For this review, take the finished solid that the model builds, in its own axes (mm). Face numbers are marked on the shaded views. A direction names the side the tool comes from. Round coordinates to 2 decimals unless told otherwise and drop trailing zeros. Loops run counter-clockwise (first coordinate to the right, second up) from the corner with the lowest first, then second, coordinate; pieces in that order, holes last.
1. To check wall thickness, follow line 1 along Y through (x, z) = (-10.5, -2); line 2 along X through (y, z) = (0.8, -0.5); line 3 along Z through (x, y) = (-11.25, 0.95). State the ranges of each line that lie inside material, in increasing order.
2. Consider section B-B on x = -6.25. State the section outline as (y, z) points, then the cut area to 3 significant figures.
3. Consider section C-C on x = -0.75. State the section outline as (y, z) points.
4. Tool access review of the marked faces 1 and 2: name each direction out of +Z, -Z, +X, -X, +Y, -Y from which nothing blocks a thin tool from reaching the whole face with its end or side.
5. Consider section A-A on z = -8. State the section outline as (x, y) points, then the cut area to 3 significant figures.
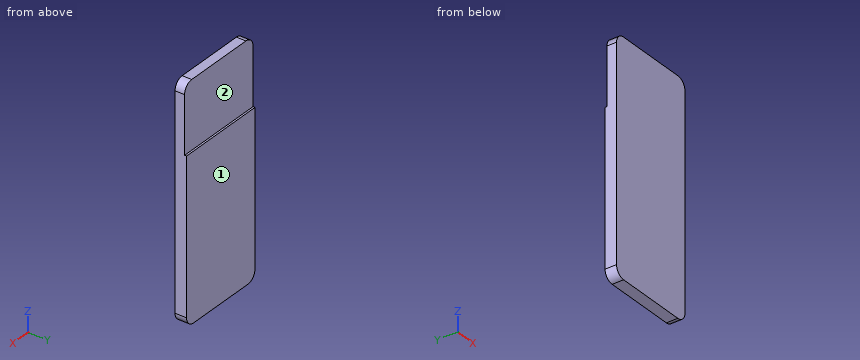
Autodesk Inventor part; units mm, degrees
ref_plane "YZ Plane" through (0, 0, 0) normal (1, 0, 0) x (0, 1, 0)
ref_plane "XZ Plane" through (0, 0, 0) normal (0, 1, 0) x (-1, 0, 0)
ref_plane "XY Plane" through (0, 0, 0) normal (0, 0, 1) x (1, 0, 0)
sketch "Sketch1" plane through (0, 0, 0) normal (0, 1, 0) x (-1, 0, 0)
  line L0 (1.27, 0) -> (10.922, 0)
  line L1 (12.192, -1.27) -> (12.192, -29.21)
  line L2 (10.922, -30.48) -> (1.27, -30.48)
  line L3 (0, -29.21) -> (0, -1.27)
  arc A0 (12.192, -1.27) -> (10.922, 0) centre (10.922, -1.27) ccw
  arc A1 (1.27, 0) -> (0, -1.27) centre (1.27, -1.27) ccw
  arc A2 (0, -29.21) -> (1.27, -30.48) centre (1.27, -29.21) ccw
  arc A3 (10.922, -30.48) -> (12.192, -29.21) centre (10.922, -29.21) ccw
  point P0 (0, 0)
  point P1 (12.192, -30.48)
  point P2 (12.192, 0)
  point P3 (0, -30.48)
  dimension "d0" = 12.192
  dimension "d1" = 30.48
  dimension "d2" = 1.27
extrude "Extrusion1" add sketch "Sketch1" along normal blind 1.524
sketch "Sketch2" plane through (0, 1.524, 0) normal (0, 1, 0) x (1, 0, 0)
  line L0 (0, 1.27) -> (0, 29.21)
  line L1 (-12.192, 0) -> (0, 0)
  line L2 (0, 0) -> (0, 8.89)
  line L3 (0, 8.89) -> (-12.192, 8.89)
  line L4 (-12.192, 8.89) -> (-12.192, 0)
  arc A0 (-12.192, 1.27) -> (-10.922, 0) centre (-10.922, 1.27) ccw
  line L5 (-10.922, 0) -> (-1.27, 0) construction
  point P0 (0, 0)
  dimension "d5" = 8.89
  dimension "d6" = 12.192
  dimension "d7" = 9.652
extrude "Extrusion2" cut sketch "Sketch2" against normal blind 0.254
properties part number "Adafruit-MicroLipoBatteryCharger"
Resolved:
1. line 1: y = 0 to 1.27
1. line 2: x = -11.93 to -0.26
1. line 3: z = -30.44 to -0.04
2. outline: (0, -30.48) - (1.52, -30.48) - (1.52, -8.89) - (1.27, -8.89) - (1.27, 0) - (0, 0) - close
2. area: 44.2 mm2
3. outline: (0, -30.37) - (1.52, -30.37) - (1.52, -8.89) - (1.27, -8.89) - (1.27, -0.11) - (0, -0.11) - close
4. face 1: +Z, -Z, +X, -X, +Y
4. face 2: +Z, +X, -X, +Y
5. outline: (-12.19, 0) - (0, 0) - (0, 1.27) - (-12.19, 1.27) - close
5. area: 15.5 mm2
